Verification items for the finished model (mm, model axes). A direction names the side the tool comes from. Give positions to 0.01 mm unless a question says otherwise; leave off trailing zeros. Write each loop counter-clockwise with the first axis right and the second up, starting at its lowest first coordinate (ties: lowest second). Pieces come first, ordered by that corner, then holes. Notation, with made-up numbers: M 77,8 L 81,8 A37 ccw 81,45 Z; hole C 18,-13 d3. An arc over 180 degrees is marked long. Answer as a JSON object with one key per item and string values.
```python
from build123d import *

# Parameters (mm, degrees)
SKETCH1_R           = 2.8448
SKETCH1_R_2         = 2.999999969
BOSS_EXTRUDE1_DEPTH = 4.4704
SKETCH2_R           = 3.2512
CUT_EXTRUDE1_DEPTH  = 1.143
CUT_EXTRUDE2_DEPTH  = 2.9972
SKETCH5_R           = 1.651
CUT_EXTRUDE3_DEPTH  = 38.18359042
SCALE1_SCALE        = 0.6


with BuildPart() as part:
    # Sketch1 → Boss-Extrude1 (new body)
    with BuildSketch(Plane(origin=(0, 0, 0), x_dir=(0, 0, -1), z_dir=(1, 0, 0))):
        with BuildLine():
            Line((0, 4.000000128), (20.485599872, 4.000000128))
            ThreePointArc((20.485599872, 4.000000128), (21.895853546, 4.584146326), (22.479999744, 5.9944))
            Line((22.479999744, 5.9944), (33.922199872, 5.9944))
            Line((33.922199872, 5.9944), (34.912799872, 5.0038))
            Line((34.912799872, 5.0038), (34.912799872, -5.0038))
            Line((34.912799872, -5.0038), (33.922199872, -5.9944))
            Line((33.922199872, -5.9944), (22.479999744, -5.9944))
            ThreePointArc((22.479999744, -5.9944), (21.895853546, -4.584146326), (20.485599872, -4.000000128))
            Line((20.485599872, -4.000000128), (0, -4.000000128))
            ThreePointArc((0, -4.000000128), (-4.000000128, 0), (0, 4.000000128))
        make_face()
        Circle(SKETCH1_R, mode=Mode.SUBTRACT)
        with Locations((27.94, 0)):
            Circle(SKETCH1_R_2, mode=Mode.SUBTRACT)
    extrude(amount=BOSS_EXTRUDE1_DEPTH)

    # Sketch2 → Cut-Extrude1 (cut)
    with BuildSketch(Plane(origin=(4.4704, 0, 0), x_dir=(0, 0, -1), z_dir=(1, 0, 0))):
        Circle(SKETCH2_R)
    extrude(amount=-CUT_EXTRUDE1_DEPTH, mode=Mode.SUBTRACT)

    # Sketch4 → Cut-Extrude2 (cut)
    with BuildSketch(Plane(origin=(4.4704, 0, 0), x_dir=(0, 0, -1), z_dir=(1, 0, 0))):
        with BuildLine():
            Line((7.0259921, 2.54), (20.3609921, 2.54))
            ThreePointArc((20.3609921, 2.54), (22.9009921, 0), (20.3609921, -2.54))
            Line((20.3609921, -2.54), (7.0259921, -2.54))
            ThreePointArc((7.0259921, -2.54), (4.4859921, 0), (7.0259921, 2.54))
        make_face()
    extrude(amount=-CUT_EXTRUDE2_DEPTH, mode=Mode.SUBTRACT)

    # Sketch5 → Cut-Extrude3 (cut, through all)
    with BuildSketch(Plane.XZ.offset(5.9944)):
        with Locations(Location((2.2352, -27.94, 0), (0, 0, 270))):
            Circle(SKETCH5_R)
    extrude(amount=-CUT_EXTRUDE3_DEPTH, mode=Mode.SUBTRACT)


with BuildPart() as part_1:
    # Scale1: scaled about (2.030165897, 0, -18.973898941)
    add(part.part.scale(SCALE1_SCALE).moved(Location((0.812066359, 0, -7.589559576))))


solid = part_1.part
```
1) Release check for a two-part mould opening along X. For faces 4 (the face through (3.494, -2, -20)), 5 (the face through (2.134, 2.741, -20.718)), 6 (the face through (1.774, 2.535, -25.269)) record: pulls with the +X half, pulls with the -X half, needs draft (parallel to the pull), parting line crosses it, or undercut.
Completed:
{"face 4": "pulls with the +X half", "face 5": "needs draft", "face 6": "undercut"}
2) Thickness scan on L1, parallel to Z at x = 1.45, y = 0.75; L2, parallel to Z at x = 3.2, y = 0.75; L3, parallel to Z at x = 2, y = 0.75. Record the ranges inside material, lowest first.
Completed:
{"L1": "z = -28.54 to -25.99, -22.72 to -9.12, -6.06 to -5.31", "L2": "z = -28.54 to -25.99, -22.72 to -21.13, -10.48 to -9.39, -5.79 to -5.31", "L3": "z = -28.54 to -25.99, -22.72 to -21.13, -10.48 to -9.12, -6.06 to -5.31"}
3) Go/stop test with flat-tipped pins: pin 1 (1.2 mm diameter, centred on x = 2.15, z = -24.35, fed in from +Y) (3 decimals); pin 2 (1.3 mm diameter, centred on x = 2.5, z = -14, fed in from -Y); pin 3 (1 mm diameter, centred on y = 0.5, z = -20.5, fed in from +X); pin 4 (1 mm diameter, centred on x = 2, y = 1, fed in from +Z). Record where each tip stops, or that it passes through.
Completed:
{"pin 1": "passes through", "pin 2": "stops at y = -2.4", "pin 3": "stops at x = 1.7", "pin 4": "stops at z = -5.24"}
4) Section check D-D on y = 1. Record the boundary of the cut face in (x, z).
Completed:
{"outline": "M 0.81,-28.54 L 3.49,-28.54 L 3.49,-25.85 L 0.81,-25.85 Z; M 0.81,-22.86 L 3.49,-22.86 L 3.49,-20.96 L 1.7,-20.96 L 1.7,-10.66 L 3.49,-10.66 L 3.49,-9.26 L 2.81,-9.26 L 2.81,-8.97 L 0.81,-8.97 Z; M 0.81,-6.21 L 2.81,-6.21 L 2.81,-5.91 L 3.49,-5.91 L 3.49,-5.41 L 0.81,-5.41 Z"}
5) Section check A-A on y = 0. Record the boundary of the cut face in (x, z).
Completed:
{"outline": "M 0.81,-28.54 L 3.49,-28.54 L 3.49,-26.15 L 0.81,-26.15 Z; M 0.81,-22.55 L 3.49,-22.55 L 3.49,-21.33 L 1.7,-21.33 L 1.7,-10.28 L 3.49,-10.28 L 3.49,-9.54 L 2.81,-9.54 L 2.81,-9.3 L 0.81,-9.3 Z; M 0.81,-5.88 L 2.81,-5.88 L 2.81,-5.64 L 3.49,-5.64 L 3.49,-5.19 L 0.81,-5.19 Z"}
6) Access from +Z, -Z, +X, -X, +Y, -Y to the whole of each face (thin tool, end or side, straight path). Record for faces 1 (the face through (2.134, -2.76, -20.736)), 2 (the face through (3, -1.524, -16)), 3 (the face through (2, 2.4, -14)).
Completed:
{"face 1": "+Z, +X, -X, -Y", "face 2": "+X", "face 3": "+Z, +X, -X, +Y"}
7) Section check B-B on z = -8.25. Record the boundary of the cut face in (x, y).
Completed:
{"outline": "M 0.81,-2.4 L 3.49,-2.4 L 3.49,-1.84 L 2.81,-1.84 L 2.81,-1.57 L 0.81,-1.57 Z; M 0.81,1.57 L 2.81,1.57 L 2.81,1.84 L 3.49,1.84 L 3.49,2.4 L 0.81,2.4 Z"}
8) Section check C-C on z = -16. Record the boundary of the cut face in (x, y), and give its area (3 significant figures).
Completed:
{"outline": "M 0.81,-2.4 L 3.49,-2.4 L 3.49,-1.52 L 1.7,-1.52 L 1.7,1.52 L 3.49,1.52 L 3.49,2.4 L 0.81,2.4 Z", "area": "7.39 mm2"}
